```python
from build123d import *

# Parameters (mm, degrees)
SKETCH_W     = 33
SKETCH_H     = 19
PAD_DEPTH    = 25
SKETCH001_R  = 6
PAD001_DEPTH = 12
SKETCH002_R  = 2
PAD002_DEPTH = 3.6
SKETCH003_W  = 9
SKETCH003_H  = 9
PAD003_DEPTH = 23
POCKET_DEPTH = 13
CHAMFER_SIZE = 1


with BuildPart() as part:
    # Sketch → Pad (new body)
    with BuildSketch(Plane.XY):
        Rectangle(SKETCH_W, SKETCH_H)
    extrude(amount=PAD_DEPTH)

    # Sketch001 (on Face6 of Pad) → Pad001 (join)
    with BuildSketch(Plane.XY.offset(25)):
        Circle(SKETCH001_R)
    extrude(amount=PAD001_DEPTH)

    # Sketch002 (on Face8 of Pad001) → Pad002 (join)
    with BuildSketch(Plane.XY.offset(37)):
        Circle(SKETCH002_R)
    extrude(amount=PAD002_DEPTH)

    # Sketch003 (on Face10 of Pad002) → Pad003 (join)
    with BuildSketch(Plane.XY.offset(40.6)):
        Rectangle(SKETCH003_W, SKETCH003_H)
    extrude(amount=PAD003_DEPTH)

    # Sketch004 (on Face2 of Pad003) → Pocket (cut)
    with BuildSketch(Plane.XZ.offset(4.5)):
        Polygon((-4.5, 40.6), (-2.214518, 63.6), (-4.5, 63.6), align=None)
    pocket = extrude(amount=-POCKET_DEPTH, mode=Mode.SUBTRACT)

    # Mirrored: Pocket across Sketch004 V_Axis
    add(pocket.mirror(Plane(origin=(0, -4.5, 0), x_dir=(0, -1, 0), z_dir=(1, 0, 0))), mode=Mode.SUBTRACT)

    # Chamfer
    chamfer_edges = [part.edges().sort_by_distance(p)[0] for p in [
        (-3.357259, -4.5, 52.1),
        (0, -4.5, 40.6),
        (3.357259, -4.5, 52.1),
        (-4.5, 0, 40.6),
        (-3.357259, 4.5, 52.1),
        (3.357259, 4.5, 52.1),
        (0, 4.5, 40.6),
        (2.214518, 0, 63.6),
        (0, -4.5, 63.6),
        (-2.214518, 0, 63.6),
        (0, 4.5, 63.6),
        (4.5, 0, 40.6),
    ]]
    chamfer(chamfer_edges, length=CHAMFER_SIZE)


solid = part.part
```
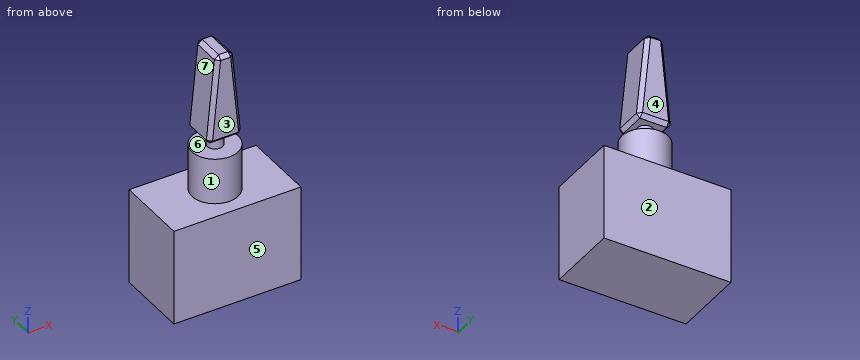
Can you work these out from the model? Positions are in its coordinate system, mm. Face numbers are marked on the shaded views. A direction names the side the tool comes from. Coordinates: 2 decimals unless noted, no trailing zeros. Order: outer loops, then holes, each group sorted by start corner. A loop starts at its lowest first (then second) coordinate and runs counter-clockwise, first axis right, second up.
1. If we section it at B-B (y = 0): Please give me the cut outline in (x, z), then the cut area to 3 significant figures.
2. If we section it at D-D (x = 8.5): Please give me the cut outline in (y, z).
3. I'm going to push flat-ended pins straight in: pin 1 (4 mm diameter, centred on x = 1, z = 40, fed in from -Y); pin 2 (1.5 mm diameter, centred on y = -2.5, z = 52, fed in from +X); pin 3 (8 mm diameter, centred on x = 4.5, y = 0.5, fed in from -Z); pin 4 (2 mm diameter, centred on x = -1.5, z = 55.5, fed in from +Y). Where does each tip first touch, or does it pass through?
4. For the marked faces 1, 2, 3 and 4, which set-ups out of +Z, -Z, +X, -X, +Y, -Y let a thin tool reach every point of the face, with its end or its side?
5. If we section it at C-C (z = 59.5): Please give me the cut outline in (x, y).
6. If we section it at A-A (x = 0): Please give me the cut outline in (y, z), then the cut area to 3 significant figures.
7. I need wall thicknesses on line 1 (Z direction, x = 6, y = -6.25); line 2 (Y direction, x = 0.5, z = 52); line 3 (Z direction, x = -4.5, y = -2.25). Which ranges of each line are inside material? Lowest first, please.
8. Thinking about a two-plate mould opening in Z: for the marked faces 5, 6 and 7, which applies, +Z half, -Z half, draft (parallel to the pull), parting line (faces both ways), or undercut?
Entries:
1. outline: (-16.5, 0) - (16.5, 0) - (16.5, 25) - (6, 25) - (6, 37) - (2, 37) - (2, 40.6) - (3.5, 40.6) - (4.4, 41.6) - (2.31, 62.6) - (1.21, 63.6) - (-1.21, 63.6) - (-2.31, 62.6) - (-4.4, 41.6) - (-3.5, 40.6) - (-2, 40.6) - (-2, 37) - (-6, 37) - (-6, 25) - (-16.5, 25) - close
1. area: 1,140 mm2
2. outline: (-9.5, 0) - (9.5, 0) - (9.5, 25) - (-9.5, 25) - close
3. pin 1: stops at y = -4.5
3. pin 2: stops at x = 3.44
3. pin 3: stops at z = 0
3. pin 4: stops at y = 4.5
4. face 1: +Z
4. face 2: +Z, -Z, +X, -X, +Y
4. face 3: +Z, +X, -X, -Y
4. face 4: +Z, +X, -X, +Y
5. outline: (-2.62, -3.5) - (-1.62, -4.5) - (1.62, -4.5) - (2.62, -3.5) - (2.62, 3.5) - (1.62, 4.5) - (-1.62, 4.5) - (-2.62, 3.5) - close
6. outline: (-9.5, 0) - (9.5, 0) - (9.5, 25) - (6, 25) - (6, 37) - (2, 37) - (2, 40.6) - (3.5, 40.6) - (4.5, 41.6) - (4.5, 62.6) - (3.5, 63.6) - (-3.5, 63.6) - (-4.5, 62.6) - (-4.5, 41.6) - (-3.5, 40.6) - (-2, 40.6) - (-2, 37) - (-6, 37) - (-6, 25) - (-9.5, 25) - close
6. area: 838 mm2
7. line 1: z = 0 to 25
7. line 2: y = -4.5 to 4.5
7. line 3: z = 0 to 37
8. face 5: draft
8. face 6: undercut
8. face 7: +Z half
